Model file for the job. Use its own axes, mm. Face numbers are marked on the shaded views. A direction names the side the tool comes from. Round coordinates to 2 decimals unless told otherwise and drop trailing zeros. Order: outer loops, then holes, each group sorted by start corner. A loop starts at its lowest first (then second) coordinate and runs counter-clockwise, first axis right, second up. Notation, with made-up numbers: (61.25, -9) - (106.25, -9) arc R33 ccw to (106.25, 20) - close; hole circle Ø4 at (84.5, 19.5). An arc over 180 degrees is marked (long way). Use one line per item in the form item = value.
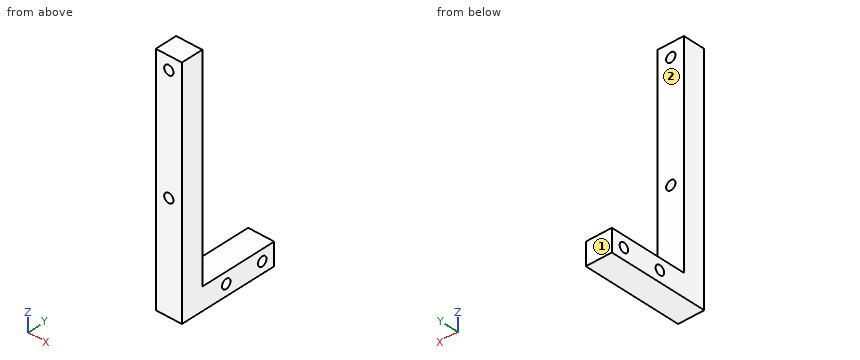
from build123d import *

# Parameters (mm, degrees)
SKETCH1_R           = 1.775
BOSS_EXTRUDE1_DEPTH = 10
SKETCH2_R           = 1.775
CUT_EXTRUDE1_DEPTH  = 65.392818275


with BuildPart() as part:
    # Sketch1 → Boss-Extrude1 (new body)
    with BuildSketch(Plane(origin=(0, 0, 0), x_dir=(0, 0, -1), z_dir=(1, 0, 0))):
        Polygon((-56.093092672, 4.635278297), (25.406907328, 4.635278297), (25.406907328, 34.635278297), (33.906907328, 34.635278297), (33.906907328, -3.864721703), (-56.093092672, -3.864721703), align=None)
        with Locations((29.656907328, 14.635278297)):
            Circle(SKETCH1_R, mode=Mode.SUBTRACT)
        with Locations((29.656907328, 29.635278297)):
            Circle(SKETCH1_R, mode=Mode.SUBTRACT)
    extrude(amount=BOSS_EXTRUDE1_DEPTH)

    # Sketch2 → Cut-Extrude1 (cut, through all)
    with BuildSketch(Plane(origin=(0, 4.635278297, 0), x_dir=(1, 0, 0), z_dir=(0, 1, 0))):
        with Locations(Location((5, -51.093092672, 0), (0, 0, 270))):
            Circle(SKETCH2_R)
        with Locations(Location((5, -7.093092672, 0), (0, 0, 270))):
            Circle(SKETCH2_R)
    extrude(amount=-CUT_EXTRUDE1_DEPTH, mode=Mode.SUBTRACT)


solid = part.part
(1) Slice it at C-C on z = 34. Give the cut face in (x, y), then the cut area to 3 significant figures.
Report:
outline = (0, -3.86) - (10, -3.86) - (10, 4.64) - (0, 4.64) - close
area = 85.0 mm2
(2) Slice it at D-D on y = 20.5. Give the cut face in (x, z), then the cut area to 3 significant figures.
Report:
outline = (0, -33.91) - (10, -33.91) - (10, -25.41) - (0, -25.41) - close
area = 85.0 mm2
(3) Slice it at B-B on x = 5. Give the cut face in (y, z) (3 decimals), then the cut area to 3 significant figures.
Report:
outline = (-3.865, -33.907) - (34.635, -33.907) - (34.635, -25.407) - (4.635, -25.407) - (4.635, 5.318) - (-3.865, 5.318) - close; (-3.865, 8.868) - (4.635, 8.868) - (4.635, 49.318) - (-3.865, 49.318) - close; (-3.865, 52.868) - (4.635, 52.868) - (4.635, 56.093) - (-3.865, 56.093) - close; hole circle Ø3.55 at (14.635, -29.657); hole circle Ø3.55 at (29.635, -29.657)
area = 940 mm2
(4) Pin check, flat tips, straight feed: pin 1 (2 mm diameter, centred on x = 5.5, z = 33.5, fed in from +Y); pin 2 (5.5 mm diameter, centred on x = 5, z = 51.09, fed in from -Y); pin 3 (3 mm diameter, centred on x = 5, z = 7.09, fed in from +Y). Stop position of each tip, or through.
Report:
pin_1 = 4.64
pin_2 = -3.86
pin_3 = through
(5) Slice it at A-A on y = 3. Give the cut face in (x, z) (3 decimals), then the cut area to 3 significant figures.
Report:
outline = (0, -33.907) - (10, -33.907) - (10, 56.093) - (0, 56.093) - close; hole circle Ø3.55 at (5, 7.093); hole circle Ø3.55 at (5, 51.093)
area = 880 mm2
(6) Probe probe 1 along Z at (x, y) = (3.5, 9); probe 2 along Y at (x, z) = (9, 48.5). List the from-to ranges inside material, lowest first. Write a range as [from, to].
Report:
probe_1 = [-33.91, -25.41]
probe_2 = [-3.86, 4.64]
(7) Tool access for the marked faces 1 and 2: list every direction of +Z, -Z, +X, -X, +Y, -Y with a clear straight run to the whole face (end or side of a thin tool).
Report:
face_1 = +Z, -Z, +X, -X, +Y
face_2 = +Z, +X, -X, +Y
